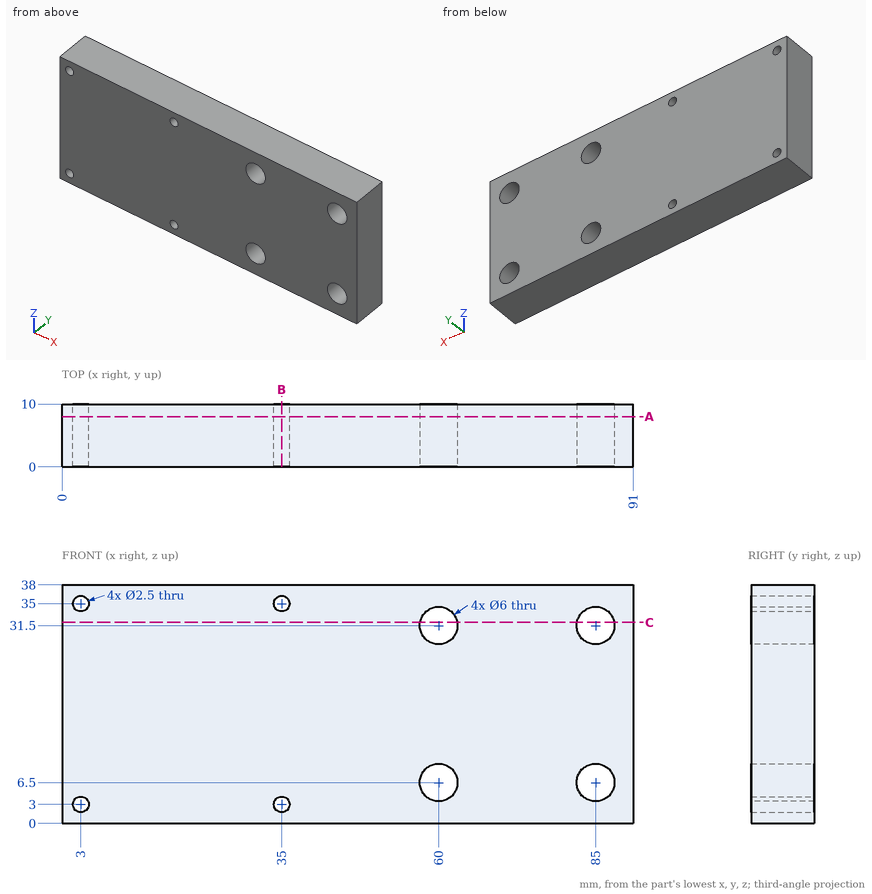
Could you check a few things on this drawing? It's one solid part, dimensions in mm from its lowest x, y, z. Round coordinates to 2 decimals unless told otherwise and drop trailing zeros. Write each loop counter-clockwise with the first axis right and the second up, starting at its lowest first coordinate (ties: lowest second). Pieces come first, ordered by that corner, then holes.
Q1. If we section it at B-B on x = 35: Write out the boundary of the cut face in (y, z), plus the area to 3 significant figures.
Q2. Will this pin go through, and if not, where does the flat tip stop? P1, Ø3, axis at x = 20, z = 10, coming from the -Y side.
Q3. If we section it at C-C on z = 32: Write out the boundary of the cut face in (x, y).
Q4. Please list where these lines run through material, in increasing order: probe 1 along Z at (x, y) = (85, 7.75); probe 2 along X at (y, z) = (5.5, 6.5); probe 3 along X at (y, z) = (2.5, 3).
Q5. If we section it at A-A on y = 8: Give the number of separate pieces and of enclosed holes in the cut face, plus the area to 3 significant figures.
Answer below:
1. outline: (0, 0) - (10, 0) - (10, 1.75) - (0, 1.75) - close; (0, 4.25) - (10, 4.25) - (10, 33.75) - (0, 33.75) - close; (0, 36.25) - (10, 36.25) - (10, 38) - (0, 38) - close
1. area: 330 mm2
2. P1: stops at y = 0
3. outline: (0, 0) - (57.04, 0) - (57.04, 10) - (0, 10) - close; (62.96, 0) - (82.04, 0) - (82.04, 10) - (62.96, 10) - close; (87.96, 0) - (91, 0) - (91, 10) - (87.96, 10) - close
4. probe 1: z = 0 to 3.5, 9.5 to 28.5, 34.5 to 38
4. probe 2: x = 0 to 57, 63 to 82, 88 to 91
4. probe 3: x = 0 to 1.75, 4.25 to 33.75, 36.25 to 91
5. separate pieces: 1
5. enclosed holes: 8
5. area: 3,330 mm2
